Verification items for the finished model (mm, model axes). A direction names the side the tool comes from. Coordinates: 2 decimals unless noted, no trailing zeros. Write each loop counter-clockwise with the first axis right and the second up, starting at its lowest first coordinate (ties: lowest second). Pieces come first, ordered by that corner, then holes. Notation, with made-up numbers: (48, 13.25) -> (82, 13.25) arc R24 cw to (82, 41.25) -> close; hole circle Ø6 at (7, 38). An arc over 180 degrees is marked (long way). Use a Markdown table: item, result. Add a question column.
from build123d import *

# Parameters (mm, degrees)
BOSS_EXTRUDE1_DEPTH = 19.0848469
SKETCH2_R           = 5
BOSS_EXTRUDE2_DEPTH = 15
CUT_EXTRUDE1_START  = -2
SKETCH3_R           = 5
SKETCH3_R_2         = 3
CUT_EXTRUDE1_DEPTH  = 2


with BuildPart() as part:
    # Sketch1 → Boss-Extrude1 (new body)
    with BuildSketch(Plane.XY):
        with BuildLine():
            Line((0, 2.5), (-4.330127019, 2.5))
            ThreePointArc((-4.330127019, 2.5), (0, -5), (4.330127019, 2.5))
            Line((4.330127019, 2.5), (0, 2.5))
        make_face()
    extrude(amount=BOSS_EXTRUDE1_DEPTH)

    # Sketch2 → Boss-Extrude2 (add)
    with BuildSketch(Plane.XY.offset(19.0848469)):
        with Locations(Location((0, 0, 0), (0, 0, 150))):
            Circle(SKETCH2_R)
    extrude(amount=BOSS_EXTRUDE2_DEPTH)

    # Sketch3 → Cut-Extrude1 (cut)
    with BuildSketch(Plane.XY.offset(32.0848469).offset(CUT_EXTRUDE1_START)):
        with Locations(Location((0, 0, 0), (0, 0, 150))):
            Circle(SKETCH3_R)
        Circle(SKETCH3_R_2, mode=Mode.SUBTRACT)
    extrude(amount=CUT_EXTRUDE1_DEPTH, mode=Mode.SUBTRACT)


solid = part.part
1) Gauge pin test, flat ends, axial feed: pin 1 (1 mm diameter, centred on x = -3.5, y = 3.5, fed in from -Z); pin 2 (1.5 mm diameter, centred on x = -3, z = 18, fed in from -Y); pin 3 (2 mm diameter, centred on x = -2, z = 28, fed in from -Y). Record the tip position at first contact, or that the pin passes through.
2) Thickness scan on L1, parallel to Z at x = -0.5, y = -3.75; L2, parallel to Z at x = 0.75, y = 4; L3, parallel to X at y = -4, z = 26. Record the ranges inside material, lowest first.
3) Cross-section at A-A on y = 4. Record the boundary of the cut face in (x, z).
4) Release check for a two-part mould opening along Z. For faces 1 (the face through (-1, 3, 30.085)), 2 (the face through (0, 4, 19.085)), 3 (the face through (-4.88, 1.08, 33.07)) record: released by +Z, released by -Z, zero draft, split by the parting line, or undercut.
5) Cross-section at B-B on x = 0. Record the boundary of the cut face in (y, z), then the cut area to 3 significant figures.
6) Cross-section at C-C on z = 29. Record the boundary of the cut face in (x, y).
7) Cross-section at D-D on x = 3.5. Record the boundary of the cut face in (y, z).
8) Set-up check for faces 4 (the face through (-3, 0, 31)), 5 (the face through (0, 2.5, 9)), 6 (the face through (0, 0, 34.085)): record each of +Z, -Z, +X, -X, +Y, -Y from which the full face is reachable in a straight line by a thin tool's end or side.
Returned:
| question | item | result |
|---|---|---|
| 1 | pin 1 | stops at z = 19.08 |
| 1 | pin 2 | stops at y = -4.47 |
| 1 | pin 3 | stops at y = -4.9 |
| 2 | L1 | z = 0 to 30.08, 32.08 to 34.08 |
| 2 | L2 | z = 19.08 to 30.08, 32.08 to 34.08 |
| 2 | L3 | x = -3 to 3 |
| 3 | outline | (-3, 19.08) -> (3, 19.08) -> (3, 30.08) -> (-3, 30.08) -> close; (-3, 32.08) -> (3, 32.08) -> (3, 34.08) -> (-3, 34.08) -> close |
| 4 | face 1 | undercut |
| 4 | face 2 | released by -Z |
| 4 | face 3 | zero draft |
| 5 | outline | (-5, 0) -> (2.5, 0) -> (2.5, 19.08) -> (5, 19.08) -> (5, 30.08) -> (3, 30.08) -> (3, 32.08) -> (5, 32.08) -> (5, 34.08) -> (-5, 34.08) -> (-5, 32.08) -> (-3, 32.08) -> (-3, 30.08) -> (-5, 30.08) -> close |
| 5 | area | 285 mm² |
| 6 | outline | circle Ø10 at (0, 0) |
| 7 | outline | (-3.57, 0) -> (2.5, 0) -> (2.5, 19.08) -> (3.57, 19.08) -> (3.57, 30.08) -> (-3.57, 30.08) -> close; (-3.57, 32.08) -> (3.57, 32.08) -> (3.57, 34.08) -> (-3.57, 34.08) -> close |
| 8 | face 4 | none |
| 8 | face 5 | -Z, +X, -X, +Y |
| 8 | face 6 | +Z, +X, -X, +Y, -Y |
